```python
from build123d import *

# Parameters (mm, degrees)
F0_W     = 130.175
F0_H     = 127
F0_R     = 2.54
F1_DEPTH = 1.5875
F3_D     = 3.556


with BuildPart() as f1:
    # F0 (on Front) → F1 (new body, symmetric)
    with BuildSketch(Plane.XZ):
        Rectangle(F0_W, F0_H)
        with Locations((-58.1025, -44.45)):
            Circle(F0_R, mode=Mode.SUBTRACT)
        with Locations((-58.1025, -34.925)):
            Circle(F0_R, mode=Mode.SUBTRACT)
        with Locations((58.1025, -44.45)):
            Circle(F0_R, mode=Mode.SUBTRACT)
        with Locations((58.1025, -34.925)):
            Circle(F0_R, mode=Mode.SUBTRACT)
        with Locations((-58.1025, 34.925)):
            Circle(F0_R, mode=Mode.SUBTRACT)
        with Locations((-58.1025, 44.45)):
            Circle(F0_R, mode=Mode.SUBTRACT)
        with Locations((58.1025, 34.925)):
            Circle(F0_R, mode=Mode.SUBTRACT)
        with Locations((58.1025, 44.45)):
            Circle(F0_R, mode=Mode.SUBTRACT)
    extrude(amount=F1_DEPTH, both=True)

    # F3 (through all)
    with Locations(Plane.XZ.offset(1.5875)):
        with Locations((-63.309373, 58.928127), (-63.309373, 1.778127), (-63.309373, -55.371873), (-50.609373, -61.721873), (0.190627, -61.721873), (50.990627, -61.721873), (63.309373, -55.371873), (63.309373, 1.778127), (63.309373, 58.928127)):
            Hole(F3_D / 2)


solid = f1.part
```
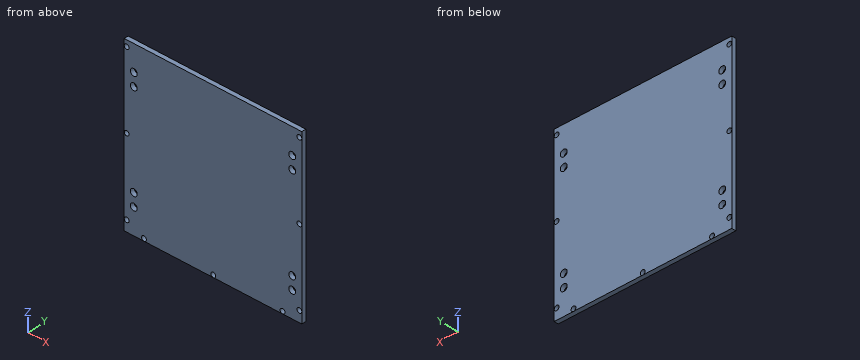
The listing builds one solid part. Answer for the finished solid, in the listing's coordinates (mm). Round coordinates to 2 decimals unless told otherwise and drop trailing zeros. Loops run counter-clockwise (first coordinate to the right, second up) from the corner with the lowest first, then second, coordinate; pieces in that order, holes last. Notation, with made-up numbers: (-22.5, 71.25) - (31.5, 71.25) arc R25 ccw to (31.5, 95.25) - close; hole circle Ø11 at (-34.75, -32). An arc over 180 degrees is marked (long way). Return JSON: item names as keys, results as strings. Group by question number.
1. Consider probe 1 along X at (y, z) = (-1.35, 0.5); probe 2 along X at (y, z) = (1.2, -33). Determine where each line is inside the solid, lowest interval first.
2. The part is cut by section B-B on y = 0.1. State how many separate pieces and enclosed holes the cut face has, then the cut area to 3 significant figures.
3. The part is cut by section A-A on z = -44.45. Determine the outline of the cut face in (x, y).
4. This flat-tipped pin is pushed along its axis until it touches: P1, Ø3, axis at x = -63.31, z = 1.78, coming from the -Y side. Where does it stop, or does it pass through?
Resolved:
{
 "1": {"probe 1": "x = -65.09 to -64.55, -62.07 to 62.07, 64.55 to 65.09", "probe 2": "x = -65.09 to -59.76, -56.45 to 56.45, 59.76 to 65.09"},
 "2": {"separate pieces": "1", "enclosed holes": "17", "area": "16,300 mm²"},
 "3": {"outline": "(-65.09, -1.59) - (-60.64, -1.59) - (-60.64, 1.59) - (-65.09, 1.59) - close; (-55.56, -1.59) - (55.56, -1.59) - (55.56, 1.59) - (-55.56, 1.59) - close; (60.64, -1.59) - (65.09, -1.59) - (65.09, 1.59) - (60.64, 1.59) - close"},
 "4": {"P1": "passes through"}
}
